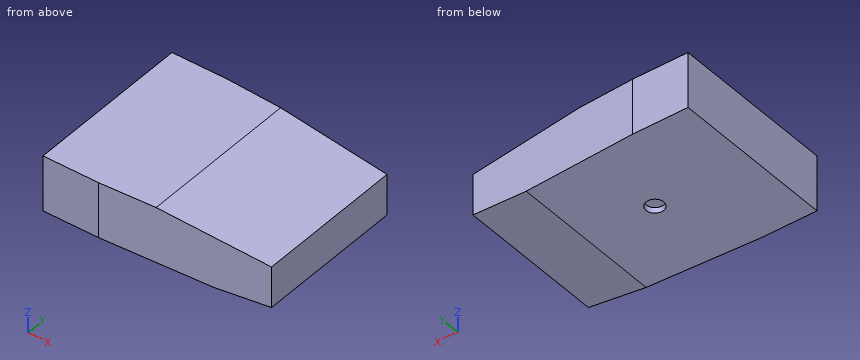
```python
from build123d import *

# Parameters (mm, degrees)
SKETCH_1_W          = 200
SKETCH_1_H          = 50
EXTRUDE_1_DEPTH     = 75
CHAMFER_1_SIZE      = 100
CHAMFER_1_SIZE2     = 8.748866353
CHAMFER_2_SIZE      = 50
CHAMFER_2_SIZE2     = 4.374433176
CHAMFER_3_SIZE      = 150
CHAMFER_3_SIZE2     = 7.861166892
CHAMFER_4_SIZE      = 150
CHAMFER_4_SIZE2     = 7.861166892
SKETCH_2_R          = 8
CUT_EXTRUDE_1_DEPTH = 5


with BuildPart() as part:
    # 草图1 → 凸台-拉伸1 (new, symmetric)
    with BuildSketch(Plane(origin=(0, 0, 0), x_dir=(1, 0, 0), z_dir=(0, 1, 0))):
        Rectangle(SKETCH_1_W, SKETCH_1_H)
    extrude(amount=EXTRUDE_1_DEPTH, both=True)

    # 倒角1
    chamfer_1_edges = [part.edges().sort_by_distance(p)[0] for p in [
        (100, 0, 25),
    ]]
    chamfer_1_side = [part.faces().sort_by_distance(p)[0] for p in [
        (0, 0, 25),
    ]]
    chamfer(chamfer_1_edges, length=CHAMFER_1_SIZE, length2=CHAMFER_1_SIZE2, reference=chamfer_1_side[0])

    # 倒角2
    chamfer_2_edges = [part.edges().sort_by_distance(p)[0] for p in [
        (100, 0, -25),
    ]]
    chamfer_2_side = [part.faces().sort_by_distance(p)[0] for p in [
        (0, 0, -25),
    ]]
    chamfer(chamfer_2_edges, length=CHAMFER_2_SIZE, length2=CHAMFER_2_SIZE2, reference=chamfer_2_side[0])

    # 倒角3
    chamfer_3_edges = [part.edges().sort_by_distance(p)[0] for p in [
        (100, -75, -2.187216588),
    ]]
    chamfer_3_side = [part.faces().sort_by_distance(p)[0] for p in [
        (-4.049031765, -75, -0.749568205),
    ]]
    chamfer(chamfer_3_edges, length=CHAMFER_3_SIZE, length2=CHAMFER_3_SIZE2, reference=chamfer_3_side[0])

    # 倒角4
    chamfer_4_edges = [part.edges().sort_by_distance(p)[0] for p in [
        (100, 75, -2.187216588),
    ]]
    chamfer_4_side = [part.faces().sort_by_distance(p)[0] for p in [
        (-4.049031765, 75, -0.749568205),
    ]]
    chamfer(chamfer_4_edges, length=CHAMFER_4_SIZE, length2=CHAMFER_4_SIZE2, reference=chamfer_4_side[0])

    # 草图2 → 切除-拉伸1 (cut)
    with BuildSketch(Plane(origin=(0, 0, -25), x_dir=(-1, 0, 0), z_dir=(0, 0, -1))):
        with Locations((12, 0)):
            Circle(SKETCH_2_R)
    extrude(amount=-CUT_EXTRUDE_1_DEPTH, mode=Mode.SUBTRACT)


solid = part.part
```
CAD build for the part. Positions are in the model's coordinates, mm. Coordinates: 2 decimals unless noted, no trailing zeros. Write each loop counter-clockwise with the first axis right and the second up, starting at its lowest first coordinate (ties: lowest second). Pieces come first, ordered by that corner, then holes. Notation, with made-up numbers: (74, 44) -> (84, 44) arc R16 ccw to (84, 52) -> close; hole circle Ø4 at (32, 81.5). An arc over 180 degrees is marked (long way). Use CSV: the item, a comma, the result in double quotes. Start each with the question number.
Item 1: Wall check: probe 1 along Y at (x, z) = (-12, -21.6); probe 2 along Z at (x, y) = (87, -55); probe 3 along Z at (x, y) = (10.5, -62). Give the ranges that are in metal, low to high.
Item 2: Band-saw the part on D-D, the plane x = 47.5. Write the cut outline in (y, z), plus the area to 3 significant figures.
Item 3: Drop flat-ended pins along their axis: P1, Ø5, axis at x = -9.5, y = 0, coming from the -Z side; P2, Ø2, axis at x = 60.5, y = -56.5, coming from the +Z side; P3, Ø2, axis at x = -29.5, z = 14.5, coming from the +Y side. Give the stop position or say it passes through.
Item 4: Band-saw the part on C-C, the plane x = -12. Write the cut outline in (y, z).
Item 5: Band-saw the part on B-B, the plane y = -54. Write the cut outline in (x, z), plus the area to 3 significant figures.
Item 6: Band-saw the part on A-A, the plane z = -11. Write the cut outline in (x, y).
Response values:
1,probe 1,"y = -73.01 to -8, 8 to 73.01"
1,probe 2,"z = -21.76 to 17.39"
1,probe 3,"z = -25 to 24.08"
2,outline,"(-69.89, -25) -> (69.89, -25) -> (69.89, 20.84) -> (-69.89, 20.84) -> close"
2,area,"6,410 mm2"
3,P1,"stops at z = -20"
3,P2,"stops at z = 19.79"
3,P3,"stops at y = 73.98"
4,outline,"(-73.01, -25) -> (-8, -25) -> (-8, -20) -> (8, -20) -> (8, -25) -> (73.01, -25) -> (73.01, 25) -> (-73.01, 25) -> close"
5,outline,"(-100, -25) -> (50, -25) -> (100, -20.63) -> (100, 16.25) -> (0, 25) -> (-100, 25) -> close"
5,area,"9,450 mm2"
6,outline,"(-100, -75) -> (-50, -75) -> (100, -67.14) -> (100, 67.14) -> (-50, 75) -> (-100, 75) -> close"
